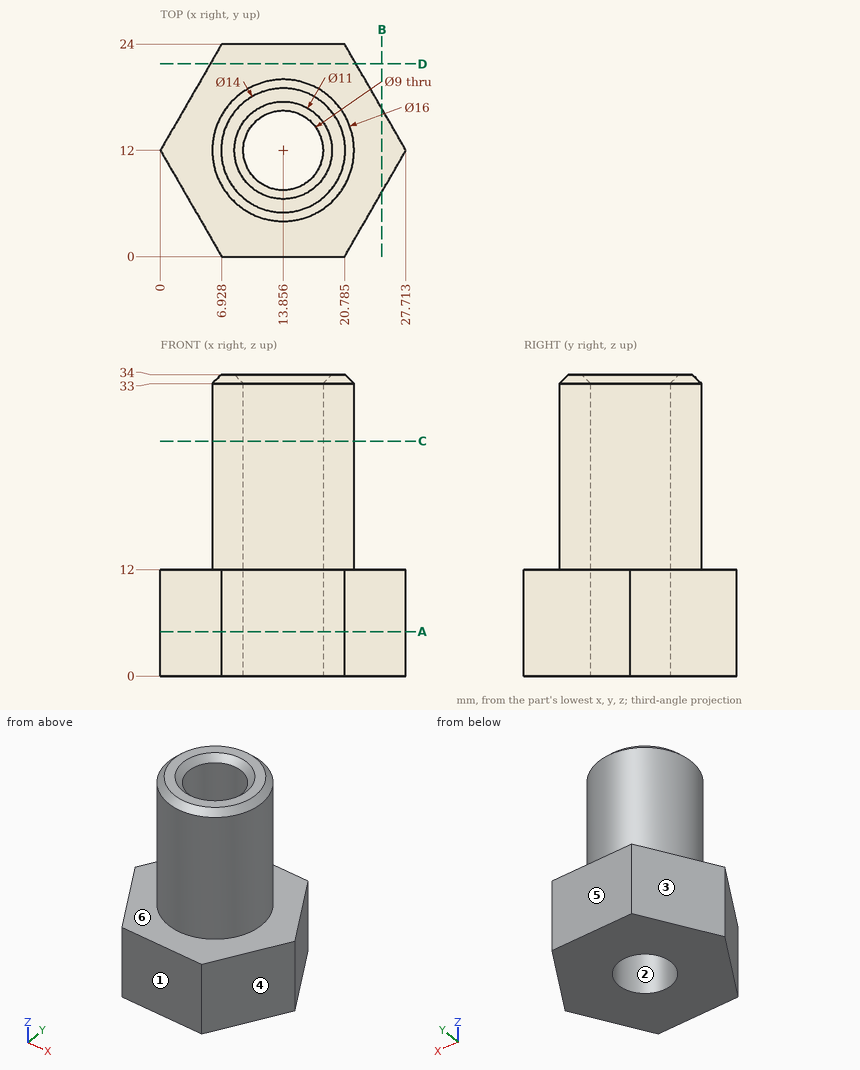
The drawing under review shows one solid part. Ordinate dimensions are in mm from its lowest x, y, z. A direction names the side the tool comes from. Give positions to 0.01 mm unless a question says otherwise; leave off trailing zeros. Order: outer loops, then holes, each group sorted by start corner. A loop starts at its lowest first (then second) coordinate and runs counter-clockwise, first axis right, second up. Notation, with made-up numbers: M 15,26 L 32,26 A24 cw 32,61 Z; hole C 65.25,-24.5 d7. An arc over 180 degrees is marked long. Answer in a Markdown table with one row per item. Add a question column.
1. Machinability: for the marked faces 5 and 6, which of the approach directions +Z, -Z, +X, -X, +Y, -Y give a long, thin tool a straight path to every point of the face, cutting with its end or side? Answer none if there is none.
2. To check wall thickness, follow line 1 along Y through (x, z) = (13.75, 18); line 2 along X through (y, z) = (12.25, 28); line 3 along Z through (x, y) = (4.5, 12). State the ranges of each line that lie inside material, in increasing order.
3. Add section B-B on x = 25. State the section outline as (y, z) points, plus the area to 3 significant figures.
4. Add section A-A on z = 5. State the section outline as (x, y) points (1 decimal), plus the area to 3 significant figures.
5. Add section C-C on z = 26.5. State the section outline as (x, y) points.
6. Mouldability with a two-part tool opening along X and no side actions: class the marked faces 1, 2, 3 and 4 as released by +X, released by -X, zero draft, split by the parting line, or undercut.
7. For pin 1 Ø2 at (x, y) = (24.5, 6) entering from +Z; pin 2 Ø5 at (y, z) = (16, 16) entering from +X (1 decimal); pin 3 Ø12 at (y, z) = (11.5, 21.5) entering from +X, all flat-tipped, find the tip position at first contact; note any pin that passes through.
8. Add section D-D on y = 21.75. State the section outline as (x, z) points.
The answers:
| question | item | result |
|---|---|---|
| 1 | face 5 | +Z, -Z, +X, -X, +Y |
| 1 | face 6 | +Z |
| 2 | line 1 | 4 to 7.5, 16.5 to 20 |
| 2 | line 2 | 5.86 to 9.36, 18.35 to 21.85 |
| 2 | line 3 | 0 to 12 |
| 3 | outline | M 7.3,0 L 16.7,0 L 16.7,12 L 7.3,12 Z |
| 3 | area | 113 mm2 |
| 4 | outline | M 0,12 L 6.9,0 L 20.8,0 L 27.7,12 L 20.8,24 L 6.9,24 Z; hole C 13.9,12 d9 |
| 4 | area | 435 mm2 |
| 5 | outline | C 13.86,12 d16; hole C 13.86,12 d9 |
| 6 | face 1 | zero draft |
| 6 | face 2 | undercut |
| 6 | face 3 | released by -X |
| 6 | face 4 | released by +X |
| 7 | pin 1 | z = 12 |
| 7 | pin 2 | x = 21.7 |
| 7 | pin 3 | x = 21.86 |
| 8 | outline | M 5.63,0 L 22.08,0 L 22.08,12 L 5.63,12 Z |
